from build123d import *

# Parameters (mm, degrees)
F0_R     = 27.5
F1_DEPTH = 120
F2_T     = -2.5
F3_W     = 10.565266
F3_H     = 9.187184
F4_DEPTH = 27.501


with BuildPart() as f1:
    # F0 (on Top) → F1 (new body)
    with BuildSketch(Plane.XY):
        Circle(F0_R)
    extrude(amount=F1_DEPTH)

    # F2
    f2_openings = [f1.faces().sort_by_distance(p)[0] for p in [
        (0, 0, 120),
    ]]
    offset(amount=F2_T, openings=f2_openings)

    # F3 (on Right) → F4 (cut, through all)
    with BuildSketch(Plane.YZ):
        with Locations((2e-06, 40.653296)):
            Rectangle(F3_W, F3_H)
    extrude(amount=-F4_DEPTH, mode=Mode.SUBTRACT)


solid = f1.part
Could you check a few things on this model? Use its own coordinates, in mm. A direction names the side the tool comes from. Give positions to 0.01 mm unless a question says otherwise; leave off trailing zeros. Loops run counter-clockwise (first coordinate to the right, second up) from the corner with the lowest first, then second, coordinate; pieces in that order, holes last. Notation, with made-up numbers: M -37,74 L -27,74 A9 ccw -27,87 Z; hole C 76,8.5 d8. An arc over 180 degrees is marked long. Answer as a JSON object with one key per item and string values.
Q1. If we mould it in two halves opening along Z, with no side actions, what happens to faces 1 (the flat face through (12.1, -22.3, 120)), 2 (the flat face through (-26, 0, 45.247)), 3 (the cylindrical face through (23.846, 7.509, 60.428))? For each: pulls with the +Z half, pulls with the -Z half, needs draft (parallel to the pull), parting line crosses it, or undercut.
Values found:
{"face 1": "pulls with the +Z half", "face 2": "undercut", "face 3": "needs draft"}
Q2. For faces 4 (the cylindrical face through (-5.961, -26.846, 59.16)), 5 (the flat face through (0, 0, 2.5)), 6 (the flat face through (-26, -5.283, 41)), which set-ups out of +Z, -Z, +X, -X, +Y, -Y let a thin tool reach every point of the face, with its end or its side?
Values found:
{"face 4": "+Z, -Z", "face 5": "+Z", "face 6": "-X"}
Q3. If I drill on probe 1 along Y at (x, z) = (0, 62); probe 2 along Z at (x, y) = (22.5, 6), over which ranges is the centre line in solid material (lowest first)? Write a range as [from, to].
Values found:
{"probe 1": "y = [-27.5, -25], [25, 27.5]", "probe 2": "z = [0, 2.5]"}
Q4. For P1, Ø8, axis at y = -9, z = 47, coming from the -X side; P2, Ø0.8, axis at x = -25.5, z = 39.5, coming from the -Y side; P3, Ø2, axis at x = -16.5, z = 73.5, coming from the +Y side; P4, Ø1, axis at x = -13, y = -12.5, coming from the -Z side, each with a flat end and sliding along its axis, tell me the tip position at first contact or that it passes through.
Values found:
{"P1": "stops at x = -27.04", "P2": "stops at y = -11.24", "P3": "stops at y = 22.72", "P4": "stops at z = 0"}
Q5. Suppose I cut it at C-C, the plane z = 62. List the corners of the cut face in (x, y) for me.
Values found:
{"outline": "C 0,0 d55; hole C 0,0 d50"}
Q6. Suppose I cut it at A-A, the plane y = 0. List the corners of the cut face in (x, z) for me, plus the area to 3 significant figures.
Values found:
{"outline": "M -27.5,0 L 27.5,0 L 27.5,120 L 25,120 L 25,2.5 L -25,2.5 L -25,36.06 L -27.5,36.06 Z; M -27.5,45.25 L -25,45.25 L -25,120 L -27.5,120 Z", "area": "702 mm²"}
Q7. Suppose I cut it at B-B, the plane x = 0. List the corners of the cut face in (y, z) for me.
Values found:
{"outline": "M -27.5,0 L 27.5,0 L 27.5,120 L 25,120 L 25,2.5 L -25,2.5 L -25,120 L -27.5,120 Z"}
Q8. Suppose I cut it at D-D, the plane y = 16. List the corners of the cut face in (x, z) for me, plus the area to 3 significant figures.
Values found:
{"outline": "M -22.37,0 L 22.37,0 L 22.37,120 L 19.21,120 L 19.21,2.5 L -19.21,2.5 L -19.21,120 L -22.37,120 Z", "area": "854 mm²"}
